Work out the finished part from the listing and answer in its coordinate system (mm). A direction names the side the tool comes from. Coordinates: 2 decimals unless noted, no trailing zeros. Write each loop counter-clockwise with the first axis right and the second up, starting at its lowest first coordinate (ties: lowest second). Pieces come first, ordered by that corner, then holes. Notation, with made-up numbers: (8.25, 42.5) - (66.25, 42.5) arc R21 cw to (66.25, 50.5) - close; hole circle Ø11 at (72.25, -7.75). An arc over 180 degrees is marked (long way). Answer as a JSON object with one key per item and string values. Group by question number.
from build123d import *

# Parameters (mm, degrees)
SKETCH2_R                           = 30
BOSS_EXTRUDE1_DEPTH                 = 50
SKETCH4_R                           = 30
BOSS_EXTRUDE4_DEPTH                 = 100
CUT_EXTRUDE3_REACH                  = 157.885
CUT_EXTRUDE3_END_RADIUS             = 30
SKETCH20_W                          = 60
SKETCH20_H                          = 14
SKETCH20_W_2                        = 40
SKETCH20_H_2                        = 10
CUT_EXTRUDE3_DIRECTION_2_REACH      = 157.885
CUT_EXTRUDE3_DIRECTION_2_END_RADIUS = 30
SKETCH8_R                           = 20
BOSS_EXTRUDE6_DEPTH                 = 50
CUT_EXTRUDE14_REACH                 = 209.403
CUT_EXTRUDE14_END_RADIUS            = 30
SKETCH22_W                          = 20
SKETCH22_H                          = 60
CUT_EXTRUDE16_REACH                 = 208.155
CUT_EXTRUDE16_END_RADIUS            = 30
SKETCH23_W                          = 20
SKETCH23_H                          = 75
V_0_377_DIAMETER_HOLE2_D            = 19.999999878
V_0_377_DIAMETER_HOLE2_DEPTH        = 30
V_0_377_DIAMETER_HOLE2_TIP          = 37.320507848
CUT_EXTRUDE17_REACH                 = 209.403
SKETCH26_R                          = 15


with BuildPart() as part:
    # Sketch2 → Boss-Extrude1 (new body)
    with BuildSketch(Plane.XY):
        Circle(SKETCH2_R)
    extrude(amount=-BOSS_EXTRUDE1_DEPTH)

    # Sketch4 → Boss-Extrude4 (add)
    with BuildSketch(Plane(origin=(0, 0, -50), x_dir=(-1, 0, 0), z_dir=(0, 0, -1))):
        with Locations(Location((0, 0, 0), (0, 0, 180))):
            Circle(SKETCH4_R)
    extrude(amount=BOSS_EXTRUDE4_DEPTH)

    # Cut-Sweep1: sweep along a curve in space
    with BuildLine() as cut_sweep1_path:
        ThreePointArc((30, 0, 0), (21.213203436, 21.213203436, 0), (0, 30, 0))
        ThreePointArc((0, 30, 0), (-21.213203436, 21.213203436, 0), (-30, 0, 0))
        ThreePointArc((-30, 0, 0), (-21.213203436, -21.213203436, 0), (0, -30, 0))
        ThreePointArc((0, -30, 0), (21.213203436, -21.213203436, 0), (30, 0, 0))
    # Sketch11 → Cut-Sweep1 (sweep, cut)
    with BuildSketch(Plane(origin=(0, 0, 0), x_dir=(0, 0, -1), z_dir=(1, 0, 0))):
        Polygon((0, 15), (50, 30), (0, 30), align=None)
    sweep(path=cut_sweep1_path.line, mode=Mode.SUBTRACT)

    # Cut-Extrude3: up to this cylinder (the profile starts inside it)
    cut_extrude3_end = Plane(origin=(0, 0, -90), z_dir=(0, 0, 1)) * Cylinder(CUT_EXTRUDE3_END_RADIUS, 376.77, mode=Mode.PRIVATE)
    # Sketch20 → Cut-Extrude3 (cut, up to the surface)
    with BuildSketch(Plane(origin=(0, 0, 0), x_dir=(0, 0, -1), z_dir=(1, 0, 0)), mode=Mode.PRIVATE) as cut_extrude3_sk1:
        with Locations((90, 23)):
            Rectangle(SKETCH20_W, SKETCH20_H)
    cut_extrude3_tool1 = extrude(cut_extrude3_sk1.sketch, amount=-CUT_EXTRUDE3_REACH, mode=Mode.PRIVATE) & cut_extrude3_end
    add(cut_extrude3_tool1.solids().sort_by_distance((0, 23, -90))[0], mode=Mode.SUBTRACT)
    # Sketch20 → Cut-Extrude3 (cut, up to the surface)
    with BuildSketch(Plane(origin=(0, 0, 0), x_dir=(0, 0, -1), z_dir=(1, 0, 0)), mode=Mode.PRIVATE) as cut_extrude3_sk2:
        with Locations((90, -25)):
            Rectangle(SKETCH20_W_2, SKETCH20_H_2)
    cut_extrude3_tool2 = extrude(cut_extrude3_sk2.sketch, amount=-CUT_EXTRUDE3_REACH, mode=Mode.PRIVATE) & cut_extrude3_end
    add(cut_extrude3_tool2.solids().sort_by_distance((0, -25, -90))[0], mode=Mode.SUBTRACT)

    # Cut-Extrude3 direction 2: up to this cylinder (the profile starts inside it)
    cut_extrude3_direction_2_end = Plane(origin=(0, 0, -90), z_dir=(0, 0, 1)) * Cylinder(CUT_EXTRUDE3_DIRECTION_2_END_RADIUS, 376.77, mode=Mode.PRIVATE)
    # Sketch20 → Cut-Extrude3 direction 2 (cut, up to the surface)
    with BuildSketch(Plane(origin=(0, 0, 0), x_dir=(0, 0, -1), z_dir=(1, 0, 0)), mode=Mode.PRIVATE) as cut_extrude3_direction_2_sk1:
        with Locations((90, 23)):
            Rectangle(SKETCH20_W, SKETCH20_H)
    cut_extrude3_direction_2_tool1 = extrude(cut_extrude3_direction_2_sk1.sketch, amount=CUT_EXTRUDE3_DIRECTION_2_REACH, mode=Mode.PRIVATE) & cut_extrude3_direction_2_end
    add(cut_extrude3_direction_2_tool1.solids().sort_by_distance((0, 23, -90))[0], mode=Mode.SUBTRACT)
    # Sketch20 → Cut-Extrude3 direction 2 (cut, up to the surface)
    with BuildSketch(Plane(origin=(0, 0, 0), x_dir=(0, 0, -1), z_dir=(1, 0, 0)), mode=Mode.PRIVATE) as cut_extrude3_direction_2_sk2:
        with Locations((90, -25)):
            Rectangle(SKETCH20_W_2, SKETCH20_H_2)
    cut_extrude3_direction_2_tool2 = extrude(cut_extrude3_direction_2_sk2.sketch, amount=CUT_EXTRUDE3_DIRECTION_2_REACH, mode=Mode.PRIVATE) & cut_extrude3_direction_2_end
    add(cut_extrude3_direction_2_tool2.solids().sort_by_distance((0, -25, -90))[0], mode=Mode.SUBTRACT)

    # Sketch8 → Boss-Extrude6 (add)
    with BuildSketch(Plane(origin=(0, 0, -150), x_dir=(-1, 0, 0), z_dir=(0, 0, -1))):
        Circle(SKETCH8_R)
    extrude(amount=BOSS_EXTRUDE6_DEPTH)

    # Cut-Extrude14: up to this cylinder (the profile starts inside it)
    cut_extrude14_end = Plane(origin=(0, 0, -30), z_dir=(0, 0, 1)) * Cylinder(CUT_EXTRUDE14_END_RADIUS, 479.806, mode=Mode.PRIVATE)
    # Sketch22 → Cut-Extrude14 (cut, up to the surface)
    with BuildSketch(Plane(origin=(0, 16, 0), x_dir=(1, 0, 0), z_dir=(0, 1, 0)), mode=Mode.PRIVATE) as cut_extrude14_sk1:
        with Locations((0, 30)):
            Rectangle(SKETCH22_W, SKETCH22_H)
    cut_extrude14_tool1 = extrude(cut_extrude14_sk1.sketch, amount=CUT_EXTRUDE14_REACH, mode=Mode.PRIVATE) & cut_extrude14_end
    add(cut_extrude14_tool1.solids().sort_by_distance((0, 16, -30))[0], mode=Mode.SUBTRACT)

    # Cut-Extrude16: up to this cylinder (the profile starts inside it)
    cut_extrude16_end = Plane(origin=(0, 0, -162.5), z_dir=(0, 0, 1)) * Cylinder(CUT_EXTRUDE16_END_RADIUS, 477.31, mode=Mode.PRIVATE)
    # Sketch23 → Cut-Extrude16 (cut, up to the surface)
    with BuildSketch(Plane(origin=(0, 10, 0), x_dir=(1, 0, 0), z_dir=(0, 1, 0)), mode=Mode.PRIVATE) as cut_extrude16_sk1:
        with Locations((0, 162.5)):
            Rectangle(SKETCH23_W, SKETCH23_H)
    cut_extrude16_tool1 = extrude(cut_extrude16_sk1.sketch, amount=CUT_EXTRUDE16_REACH, mode=Mode.PRIVATE) & cut_extrude16_end
    add(cut_extrude16_tool1.solids().sort_by_distance((0, 10, -162.5))[0], mode=Mode.SUBTRACT)

    # V (0.377) Diameter Hole2
    with Locations(Plane.XY):
        with Locations((0, 0)):
            Hole(V_0_377_DIAMETER_HOLE2_D / 2, depth=V_0_377_DIAMETER_HOLE2_DEPTH)
            with Locations((0, 0, -(V_0_377_DIAMETER_HOLE2_DEPTH + V_0_377_DIAMETER_HOLE2_TIP / 2))):  # 30° drill point
                Cone(0, V_0_377_DIAMETER_HOLE2_D / 2, V_0_377_DIAMETER_HOLE2_TIP, mode=Mode.SUBTRACT)

    # Sketch26 → Cut-Extrude17 (cut, up to next)
    with BuildSketch(Plane(origin=(0, 16, 0), x_dir=(1, 0, 0), z_dir=(0, 1, 0)), mode=Mode.PRIVATE) as cut_extrude17_sk1:
        with Locations(Location((0, 90, 0), (0, 0, 270))):
            Circle(SKETCH26_R)
    cut_extrude17_tool1 = extrude(cut_extrude17_sk1.sketch, amount=-CUT_EXTRUDE17_REACH, mode=Mode.PRIVATE) & part.part
    add(cut_extrude17_tool1.solids().sort_by_distance((0, 16, -90))[0], mode=Mode.SUBTRACT)


solid = part.part
Q1. Section B-B on z = -128 is taken. Determine the outline of the cut face in (x, y).
Q2. A tool of negligible diameter and unlimited length cuts with its end or side. For faces 5 (the face through (-16, 21, -60)), 6 (the face through (-10, 21, -41)), 7 (the face through (0.733, -19.987, -174.65)), 8 (the face through (0, 10, -163)), from which of +Z, -Z, +X, -X, +Y, -Y can it reach the whole face along a straight path? Write none if from no direction.
Q3. Section D-D on z = -65.5 is taken. Determine the outline of the cut face in (x, y).
Q4. Consider L1, parallel to Y at x = 0, z = -17.75 (3 decimals); L2, parallel to X at y = -6, z = -88; L3, parallel to X at y = -20, z = -147. Determine where each line is inside the solid, lowest interval first. Write a range as from..to.
Q5. For a pull along X with two mould halves and no side action, classify faces 1 (the face through (-4.614, -8.872, -15.21)), 2 (the face through (-10, 17, -154)), 3 (the face through (-15.2, -20, -89.7)), 4 (the face through (16.128, -25.296, -110.411)) as +X half, -X half, draft (parallel to the pull), parting line (faces both ways), or undercut.
Q6. Section A-A on z = -90 is taken. Determine the outline of the cut face in (x, y).
Q7. Section C-C on y = 26 is taken. Count the separate pieces of the cut face and the enclosed holes in it, plus the area to 3 significant figures.
Q8. Flat-ended cylindrical pins translate along their axes: pin 1 Ø3.5 at (x, y) = (-16, 21.5) entering from -Z; pin 2 Ø10 at (y, z) = (-9.5, -175.5) entering from +X; pin 3 Ø1 at (y, z) = (6, -162.5) entering from -X. Find the tip coordinate at first contact, or state that the pin passes through.
Numbers:
{
 "1": {"outline": "(-10, 10) - (-10, 28.28) arc R30 ccw (long way) to (10, 28.28) - (10, 10) - close"},
 "2": {"face 5": "+X, -X, +Y", "face 6": "+Z, +Y", "face 7": "-Z", "face 8": "-Z, +Y"},
 "3": {"outline": "(-25.38, 16) arc R30 ccw (long way) to (25.38, 16) - close; hole circle Ø0.98 at (0, 0)"},
 "4": {"L1": "y = -20.325..-10, 10..16", "L2": "x = -29.39..-14.87, 14.87..29.39", "L3": "x = -22.36..22.36"},
 "5": {"face 1": "undercut", "face 2": "undercut", "face 3": "draft", "face 4": "parting line"},
 "6": {"outline": "(-25.38, 16) arc R30 ccw to (-22.36, -20) - (-15, -20) - (-15, 16) - close; (15, -20) - (22.36, -20) arc R30 ccw to (25.38, 16) - (15, 16) - close"},
 "7": {"separate pieces": "3", "enclosed holes": "0", "area": "535 mm²"},
 "8": {"pin 1": "stops at z = -150", "pin 2": "stops at x = 19.49", "pin 3": "stops at x = -19.23"}
}
